Check sheet for the drawn part. Datum: minimum x, y, z corner. Units: mm. A direction names the side the tool comes from. Give positions to 0.01 mm unless a question says otherwise; leave off trailing zeros. Write each loop counter-clockwise with the first axis right and the second up, starting at its lowest first coordinate (ties: lowest second). Pieces come first, ordered by that corner, then holes. Notation, with made-up numbers: (68, 59.5) - (75, 59.5) arc R19 ccw to (75, 80.5) - close; hole circle Ø9 at (46.5, 44). An arc over 180 degrees is marked (long way). Use a Markdown table: item, result.
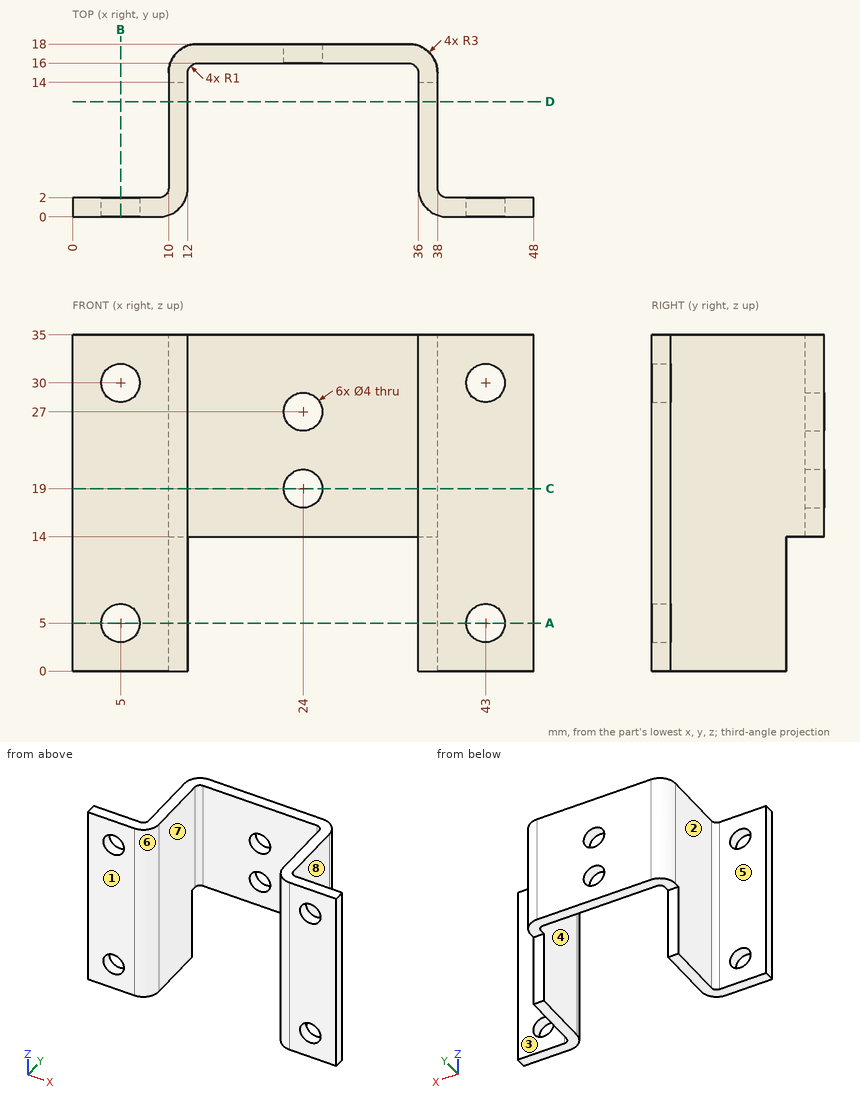
1) Material ranges on L1, parallel to Z at x = 24, y = 17.2; L2, parallel to Z at x = 5, y = 0.85; L3, parallel to X at y = 4.5, z = 28, recorded low to high. Write a range as from..to.
Working result:
| item | result |
|---|---|
| L1 | z = 14..17, 21..25, 29..35 |
| L2 | z = 0..3, 7..28, 32..35 |
| L3 | x = 10..12, 36..38 |
2) Depth check by flat-ended pin: P1, Ø5, axis at y = 11.5, z = 21, coming from the -X side; P2, Ø17, axis at x = 22.5, z = 19.5, coming from the -Y side; P3, Ø4.5, axis at x = 43, z = 5, coming from the +Y side. Enter the tip coordinate at first touch or a pass-through.
Working result:
| item | result |
|---|---|
| P1 | stops at x = 10 |
| P2 | stops at y = 16 |
| P3 | stops at y = 2 |
3) Mould release check, pull along X, two halves, no side actions. Record for the marked faces 5, 6, 7 and 8: pulls with the +X half, pulls with the -X half, needs draft (parallel to the pull), parting line crosses it, or undercut.
Working result:
| item | result |
|---|---|
| face 5 | needs draft |
| face 6 | undercut |
| face 7 | undercut |
| face 8 | pulls with the +X half |
4) Section check D-D on y = 12. Record the boundary of the cut face in (x, z), then the cut area to 3 significant figures.
Working result:
| item | result |
|---|---|
| outline | (10, 0) - (12, 0) - (12, 35) - (10, 35) - close; (36, 0) - (38, 0) - (38, 35) - (36, 35) - close |
| area | 140 mm² |
5) Section check C-C on z = 19. Record the boundary of the cut face in (x, y).
Working result:
| item | result |
|---|---|
| outline | (0, 0) - (9, 0) arc R3 ccw to (12, 3) - (12, 15) arc R1 cw to (13, 16) - (22, 16) - (22, 18) - (13, 18) arc R3 ccw to (10, 15) - (10, 3) arc R1 cw to (9, 2) - (0, 2) - close; (26, 16) - (35, 16) arc R1 cw to (36, 15) - (36, 3) arc R3 ccw to (39, 0) - (48, 0) - (48, 2) - (39, 2) arc R1 cw to (38, 3) - (38, 15) arc R3 ccw to (35, 18) - (26, 18) - close |
6) Section check A-A on z = 5. Record the boundary of the cut face in (x, y), then the cut area to 3 significant figures.
Working result:
| item | result |
|---|---|
| outline | (0, 0) - (3, 0) - (3, 2) - (0, 2) - close; (7, 0) - (9, 0) arc R3 ccw to (12, 3) - (12, 14) - (10, 14) - (10, 3) arc R1 cw to (9, 2) - (7, 2) - close; (36, 3) arc R3 ccw to (39, 0) - (41, 0) - (41, 2) - (39, 2) arc R1 cw to (38, 3) - (38, 14) - (36, 14) - close; (45, 0) - (48, 0) - (48, 2) - (45, 2) - close |
| area | 76.6 mm² |
7) Section check B-B on x = 5. Record the boundary of the cut face in (y, z).
Working result:
| item | result |
|---|---|
| outline | (0, 0) - (2, 0) - (2, 3) - (0, 3) - close; (0, 7) - (2, 7) - (2, 28) - (0, 28) - close; (0, 32) - (2, 32) - (2, 35) - (0, 35) - close |
8) Set-up check for the marked faces 1, 2, 3 and 4: record each of +Z, -Z, +X, -X, +Y, -Y from which the full face is reachable in a straight line by a thin tool's end or side.
Working result:
| item | result |
|---|---|
| face 1 | +Z, -Z, +X, -X, -Y |
| face 2 | +Z, -Z, -X, +Y |
| face 3 | +Z, -Z, +X, +Y |
| face 4 | +Z, -Z, -Y |
